Can you work these out from the model? Positions are in its coordinate system, mm. Face numbers are marked on the shaded views. A direction names the side the tool comes from. Round coordinates to 2 decimals unless told otherwise and drop trailing zeros. Loops run counter-clockwise (first coordinate to the right, second up) from the corner with the lowest first, then second, coordinate; pieces in that order, holes last. Notation, with made-up numbers: M 81.25,3.25 L 99.25,3.25 A10 cw 99.25,19.25 Z; hole C 87.5,31.5 d8. An arc over 180 degrees is marked long. Return JSON: item names as keys, results as strings.
```python
from build123d import *

# Parameters (mm, degrees)
SKETCH1_R               = 20
SKETCH1_R_2             = 6
SKETCH1_R_3             = 1.5
BOSS_EXTRUDE1_DEPTH     = 5
SKETCH2_R               = 9
SKETCH2_R_2             = 6
BOSS_EXTRUDE2_DEPTH     = 10
SKETCH3_R               = 50
SKETCH3_R_2             = 6
BOSS_EXTRUDE3_DEPTH     = 2
CUT_EXTRUDE1_START      = -2
CUT_EXTRUDE1_DEPTH      = 2
CUT_EXTRUDE2_DEPTH      = 73.284161474
CUT_EXTRUDE2_DEPTH_BACK = 73.284161474
SKETCH5_R               = 1.5


with BuildPart() as part:
    # Sketch1 → Boss-Extrude1 (new body)
    with BuildSketch(Plane.XY):
        Circle(SKETCH1_R)
        Circle(SKETCH1_R_2, mode=Mode.SUBTRACT)
        with Locations((-10.061951403, 10.061951403)):
            Circle(SKETCH1_R_3, mode=Mode.SUBTRACT)
        with Locations(Location((10.061951403, 10.061951403, 0), (0, 0, 180))):
            Circle(SKETCH1_R_3, mode=Mode.SUBTRACT)
        with Locations((10.061951403, -10.061951403)):
            Circle(SKETCH1_R_3, mode=Mode.SUBTRACT)
        with Locations(Location((-10.061951403, -10.061951403, 0), (0, 0, 180))):
            Circle(SKETCH1_R_3, mode=Mode.SUBTRACT)
    extrude(amount=BOSS_EXTRUDE1_DEPTH)

    # Sketch2 → Boss-Extrude2 (add)
    with BuildSketch(Plane.XY.offset(5)):
        Circle(SKETCH2_R)
        Circle(SKETCH2_R_2, mode=Mode.SUBTRACT)
    extrude(amount=BOSS_EXTRUDE2_DEPTH)

    # Sketch3 → Boss-Extrude3 (add)
    with BuildSketch(Plane.XY.offset(5)):
        Circle(SKETCH3_R)
        Circle(SKETCH3_R_2, mode=Mode.SUBTRACT)
    extrude(amount=BOSS_EXTRUDE3_DEPTH)

    # Sketch4 → Cut-Extrude1 (cut)
    with BuildSketch(Plane.XY.offset(7).offset(CUT_EXTRUDE1_START)):
        with BuildLine():
            Line((-7, 49.507575178), (-7, 34.507575178))
            ThreePointArc((-7, 34.507575178), (0, 27.507575178), (7, 34.507575178))
            Line((7, 34.507575178), (7, 49.507575178))
            ThreePointArc((7, 49.507575178), (0, 50), (-7, 49.507575178))
        make_face()
        with BuildLine():
            Line((49.507575178, -7), (34.507575178, -7))
            ThreePointArc((34.507575178, -7), (27.507575178, 0), (34.507575178, 7))
            Line((34.507575178, 7), (49.507575178, 7))
            ThreePointArc((49.507575178, 7), (50, 0), (49.507575178, -7))
        make_face()
    extrude(amount=CUT_EXTRUDE1_DEPTH, mode=Mode.SUBTRACT)

    # Sketch5 → Cut-Extrude2 (cut, two sides: drawn at the far end of the back side and taken through both)
    with BuildSketch(Plane(origin=(0, 0, 0), x_dir=(-1, 0, 0), z_dir=(0, 0, -1)).offset(-CUT_EXTRUDE2_DEPTH_BACK)):
        with Locations((-10.061951403, 10.061951403)):
            Circle(SKETCH5_R)
        with Locations(Location((-10.061951403, -10.061951403, 0), (0, 0, 180))):
            Circle(SKETCH5_R)
        with Locations(Location((10.061951403, 10.061951403, 0), (0, 0, 180))):
            Circle(SKETCH5_R)
        with Locations((10.061951403, -10.061951403)):
            Circle(SKETCH5_R)
    extrude(amount=CUT_EXTRUDE2_DEPTH + CUT_EXTRUDE2_DEPTH_BACK, mode=Mode.SUBTRACT)


solid = part.part
```
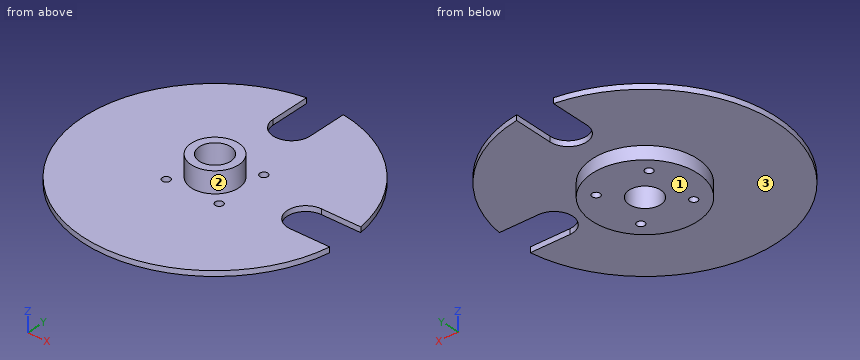
Q1. I'm going to push flat-ended pins straight in: pin 1 Ø1.5 at (y, z) = (36, 8.5) entering from -X; pin 2 Ø1 at (y, z) = (11, 3) entering from +X; pin 3 Ø1 at (x, z) = (41, 6.5) entering from +Y; pin 4 Ø0.6 at (x, z) = (41, 6) entering from -Y. Where does each tip first touch, or does it pass through?
Results:
{"pin 1": "passes through", "pin 2": "stops at x = 17.02", "pin 3": "stops at y = 29.32", "pin 4": "stops at y = -29.04"}
Q2. Suppose I cut it at C-C, the plane z = 1.5. Please give me the cut outline in (x, y), plus the area to 3 significant figures.
Results:
{"outline": "C 0,0 d40; hole C -10.06,-10.06 d3; hole C -10.06,10.06 d3; hole C 0,0 d12; hole C 10.06,-10.06 d3; hole C 10.06,10.06 d3", "area": "1,120 mm2"}
Q3. On a 3-axis mill with a long thin cutter (end or side, diameter ignored), from which of +Z, -Z, +X, -X, +Y, -Y can I reach the whole of each face in a straight line? I mean the marked faces 1, 2 and 3. Say none if no direction works.
Results:
{"face 1": "-Z, +X, -X, +Y, -Y", "face 2": "+Z", "face 3": "-Z"}
Q4. Suppose I cut it at D-D, the plane y = -17. Please give me the cut outline in (x, z).
Results:
{"outline": "M -47.02,5 L -10.54,5 L -10.54,0 L 10.54,0 L 10.54,5 L 47.02,5 L 47.02,7 L -47.02,7 Z"}
Q5. If I drill on line 1 along X through (y, z) = (-11, 4); line 2 along Z through (x, y) = (2, -23.5); line 3 along Z through (x, y) = (-2.5, 18.5), over which ranges is the centre line in solid material (lowest first)?
Results:
{"line 1": "x = -16.7 to -11.23, -8.89 to 8.89, 11.23 to 16.7", "line 2": "z = 5 to 7", "line 3": "z = 0 to 7"}
Q6. Suppose I cut it at A-A, the plane x = 0. Please give me the cut outline in (y, z), plus the area to 3 significant figures.
Results:
{"outline": "M -50,5 L -20,5 L -20,0 L -6,0 L -6,15 L -9,15 L -9,7 L -50,7 Z; M 6,0 L 20,0 L 20,5 L 27.51,5 L 27.51,7 L 9,7 L 9,15 L 6,15 Z", "area": "319 mm2"}
